from build123d import *

# Parameters (mm, degrees)
CROQUIS1_R              = 15
SALIENTE_EXTRUIR1_DEPTH = 4
CROQUIS2_R              = 23.75
SALIENTE_EXTRUIR2_DEPTH = 26
CROQUIS3_R              = 2.5
CORTAR_EXTRUIR1_DEPTH   = 40
CORTAR_EXTRUIR3_START   = -3
CROQUIS4_R              = 20.840702769
CROQUIS4_R_2            = 9.281745818
CORTAR_EXTRUIR3_DEPTH   = 19


with BuildPart() as part:
    # Croquis1 → Saliente-Extruir1 (new body)
    with BuildSketch(Plane(origin=(0, 0, 0), x_dir=(1, 0, 0), z_dir=(0, 1, 0))):
        with Locations(Location((0, 0, 0), (0, 0, 270))):
            Circle(CROQUIS1_R)
    extrude(amount=SALIENTE_EXTRUIR1_DEPTH)

    # Croquis2 → Saliente-Extruir2 (add)
    with BuildSketch(Plane(origin=(0, 4, 0), x_dir=(1, 0, 0), z_dir=(0, 1, 0))):
        with Locations(Location((0, 0, 0), (0, 0, 90))):
            Circle(CROQUIS2_R)
    extrude(amount=SALIENTE_EXTRUIR2_DEPTH)

    # Croquis3 → Cortar-Extruir1 (cut)
    with BuildSketch(Plane(origin=(0, 30, 0), x_dir=(1, 0, 0), z_dir=(0, 1, 0))):
        with Locations(Location((0, 0, 0), (0, 0, 270))):
            Circle(CROQUIS3_R)
    extrude(amount=-CORTAR_EXTRUIR1_DEPTH, mode=Mode.SUBTRACT)

    # Croquis4 → Cortar-Extruir3 (cut)
    with BuildSketch(Plane(origin=(0, 30, 0), x_dir=(1, 0, 0), z_dir=(0, 1, 0)).offset(CORTAR_EXTRUIR3_START)):
        with Locations(Location((0, 0, 0), (0, 0, 270))):
            Circle(CROQUIS4_R)
        with Locations(Location((0, 0, 0), (0, 0, 270))):
            Circle(CROQUIS4_R_2, mode=Mode.SUBTRACT)
    extrude(amount=-CORTAR_EXTRUIR3_DEPTH, mode=Mode.SUBTRACT)


solid = part.part
CAD build for the part. Positions are in the model's coordinates, mm. A direction names the side the tool comes from. Round coordinates to 2 decimals unless told otherwise and drop trailing zeros. Write each loop counter-clockwise with the first axis right and the second up, starting at its lowest first coordinate (ties: lowest second). Pieces come first, ordered by that corner, then holes. Notation, with made-up numbers: M -30,-7 L -19,-7 A15 ccw -19,16 Z; hole C -14.75,-29 d11. An arc over 180 degrees is marked long. Use a Markdown table: item, result. Add a question column.
1. Slice it at C-C on y = 15. Give the cut face in (x, z).
2. Flat gauge pins, fed straight in: P1, Ø14, axis at x = -1.5, z = 1.5, coming from the -Y side; P2, Ø8, axis at x = 13, y = 4, coming from the +Z side; P3, Ø1.5, axis at y = 5, z = 16, coming from the -X side; P4, Ø8, axis at y = 12.5, z = 8, coming from the +X side. Where does each tip first touch, or does it go through?
3. 3-axis set-ups, long thin cutter, end or side, ignore diameter. For faces 5 (the face through (0, 0, 3)), 6 (the face through (0, 4, -16)), 7 (the face through (6.273, 17.633, -6.841)): which of +Z, -Z, +X, -X, +Y, -Y reach the whole face in a straight line?
4. Slice it at A-A on x = 0. Give the cut face in (y, z), then the cut area to 3 significant figures.
5. Drill centre lines: probe 1 along X at (y, z) = (17.25, 0); probe 2 along Z at (x, y) = (2, 22.5); probe 3 along Y at (x, z) = (-15.5, 12.5). Where is each one in solid material? Low to high.
6. Slice it at D-D on x = -20. Give the cut face in (y, z).
7. Pull direction X, two halves, no side cores. Call faces 1 (the face through (0, 30, -5)), 2 (the face through (-4, 8, 9)), 3 (the face through (-2.44, 15.21, -0.54)), 4 (the face through (0.66, 1.972, -14.985)): released by +X, released by -X, zero draft, split by the parting line, or undercut.
8. Slice it at B-B on z = 0. Give the cut face in (x, y).
Reply:
| question | item | result |
|---|---|---|
| 1 | outline | C 0,0 d47.5; C 0,0 d18.56; hole C 0,0 d41.68; hole C 0,0 d5 |
| 2 | P1 | stops at y = 0 |
| 2 | P2 | stops at z = 21.98 |
| 2 | P3 | stops at x = -18.21 |
| 2 | P4 | stops at x = 23.41 |
| 3 | face 5 | +Z, -Z, +X, -X, -Y |
| 3 | face 6 | -Y |
| 3 | face 7 | none |
| 4 | outline | M 0,-15 L 4,-15 L 4,-23.75 L 30,-23.75 L 30,-2.5 L 0,-2.5 Z; M 0,2.5 L 30,2.5 L 30,23.75 L 4,23.75 L 4,15 L 0,15 Z; hole M 8,-20.84 L 27,-20.84 L 27,-9.28 L 8,-9.28 Z; hole M 8,9.28 L 27,9.28 L 27,20.84 L 8,20.84 Z |
| 4 | area | 766 mm^2 |
| 5 | probe 1 | x = -23.75 to -20.84, -9.28 to -2.5, 2.5 to 9.28, 20.84 to 23.75 |
| 5 | probe 2 | z = -23.67 to -20.74, -9.06 to -1.5, 1.5 to 9.06, 20.74 to 23.67 |
| 5 | probe 3 | y = 4 to 8, 27 to 30 |
| 6 | outline | M 4,-12.81 L 30,-12.81 L 30,12.81 L 4,12.81 Z; hole M 8,-5.86 L 27,-5.86 L 27,5.86 L 8,5.86 Z |
| 7 | face 1 | zero draft |
| 7 | face 2 | undercut |
| 7 | face 3 | undercut |
| 7 | face 4 | split by the parting line |
| 8 | outline | M -23.75,4 L -15,4 L -15,0 L -2.5,0 L -2.5,30 L -23.75,30 Z; M 2.5,0 L 15,0 L 15,4 L 23.75,4 L 23.75,30 L 2.5,30 Z; hole M -20.84,8 L -9.28,8 L -9.28,27 L -20.84,27 Z; hole M 9.28,8 L 20.84,8 L 20.84,27 L 9.28,27 Z |
